Can you work these out from the model? Positions are in its coordinate system, mm. Face numbers are marked on the shaded views. Round coordinates to 2 decimals unless told otherwise and drop trailing zeros. Loops run counter-clockwise (first coordinate to the right, second up) from the corner with the lowest first, then second, coordinate; pieces in that order, holes last. Notation, with made-up numbers: (-35.75, -27.5) -> (-25.75, -27.5) arc R26 cw to (-25.75, -3.5) -> close; hole circle Ø7 at (-31, -4). An arc over 180 degrees is marked (long way). Use a Markdown table: item, result.
from build123d import *

# Parameters (mm, degrees)
BOSS_EXTRUDE1_DEPTH = 25
BOSS_EXTRUDE2_DEPTH = 15
CUT_EXTRUDE1_REACH  = 42.894
SKETCH3_R           = 1.5
CUT_EXTRUDE2_REACH  = 42.894
SKETCH4_R           = 1.6
CUT_EXTRUDE3_DEPTH  = 41.591655546


with BuildPart() as part:
    # Sketch1 → Boss-Extrude1 (new body)
    with BuildSketch(Plane.XY):
        Polygon((0, 0), (4.128054425, 7.15), (-4.6, 7.15), (-4.6, 5.15), (0.66395281, 5.15), (-1.732050808, 1), align=None)
    extrude(amount=BOSS_EXTRUDE1_DEPTH)

    # Sketch2 → Boss-Extrude2 (add)
    with BuildSketch(Plane.XY.offset(25)):
        Polygon((4.128054425, 7.15), (0, 0), (-1.732050808, 1), (1.818653348, 7.15), align=None)
    extrude(amount=BOSS_EXTRUDE2_DEPTH)

    # Sketch3 → Cut-Extrude1 (cut, up to next)
    with BuildSketch(Plane(origin=(0, 0, 0), x_dir=(0, 0, -1), z_dir=(0.8660254037844365, -0.5000000000000039, 0)), mode=Mode.PRIVATE) as cut_extrude1_sk1:
        with Locations(Location((-37.5, 2.5, 0), (0, 0, 90))):
            Circle(SKETCH3_R)
    cut_extrude1_tool1 = extrude(cut_extrude1_sk1.sketch, amount=-CUT_EXTRUDE1_REACH, mode=Mode.PRIVATE) & part.part
    # Sketch3 → Cut-Extrude1 (cut, up to next)
    with BuildSketch(Plane(origin=(0, 0, 0), x_dir=(0, 0, -1), z_dir=(0.8660254037844365, -0.5000000000000039, 0)), mode=Mode.PRIVATE) as cut_extrude1_sk2:
        with Locations(Location((-2.5, 2.5, 0), (0, 0, 90))):
            Circle(SKETCH3_R)
    cut_extrude1_tool2 = extrude(cut_extrude1_sk2.sketch, amount=-CUT_EXTRUDE1_REACH, mode=Mode.PRIVATE) & part.part
    add(cut_extrude1_tool1.solids().sort_by_distance((1.25, 2.165064, 37.5))[0], mode=Mode.SUBTRACT)
    add(cut_extrude1_tool2.solids().sort_by_distance((1.25, 2.165064, 2.5))[0], mode=Mode.SUBTRACT)

    # Sketch4 → Cut-Extrude2 (cut, up to next)
    with BuildSketch(Plane(origin=(0, 7.15, 0), x_dir=(1, 0, 0), z_dir=(0, 1, 0)), mode=Mode.PRIVATE) as cut_extrude2_sk1:
        with Locations(Location((-0.6, -8, 0), (0, 0, 180))):
            Circle(SKETCH4_R)
    cut_extrude2_tool1 = extrude(cut_extrude2_sk1.sketch, amount=-CUT_EXTRUDE2_REACH, mode=Mode.PRIVATE) & part.part
    # Sketch4 → Cut-Extrude2 (cut, up to next)
    with BuildSketch(Plane(origin=(0, 7.15, 0), x_dir=(1, 0, 0), z_dir=(0, 1, 0)), mode=Mode.PRIVATE) as cut_extrude2_sk2:
        with Locations(Location((-0.6, -20.5, 0), (0, 0, 180))):
            Circle(SKETCH4_R)
    cut_extrude2_tool2 = extrude(cut_extrude2_sk2.sketch, amount=-CUT_EXTRUDE2_REACH, mode=Mode.PRIVATE) & part.part
    add(cut_extrude2_tool1.solids().sort_by_distance((-0.6, 7.15, 8))[0], mode=Mode.SUBTRACT)
    add(cut_extrude2_tool2.solids().sort_by_distance((-0.6, 7.15, 20.5))[0], mode=Mode.SUBTRACT)

    # Sketch5 → Cut-Extrude3 (cut, through all)
    with BuildSketch(Plane.XZ.offset(-5.15)):
        with BuildLine():
            Line((-0.6, 23.5), (-3.6, 23.5))
            Line((-3.6, 23.5), (-3.6, 17.5))
            Line((-3.6, 17.5), (-0.6, 17.5))
            ThreePointArc((-0.6, 17.5), (2.4, 20.5), (-0.6, 23.5))
        make_face()
        with BuildLine():
            Line((-0.6, 11), (-3.6, 11))
            Line((-3.6, 11), (-3.6, 5))
            Line((-3.6, 5), (-0.6, 5))
            ThreePointArc((-0.6, 5), (2.4, 8), (-0.6, 11))
        make_face()
    extrude(amount=CUT_EXTRUDE3_DEPTH, mode=Mode.SUBTRACT)


solid = part.part
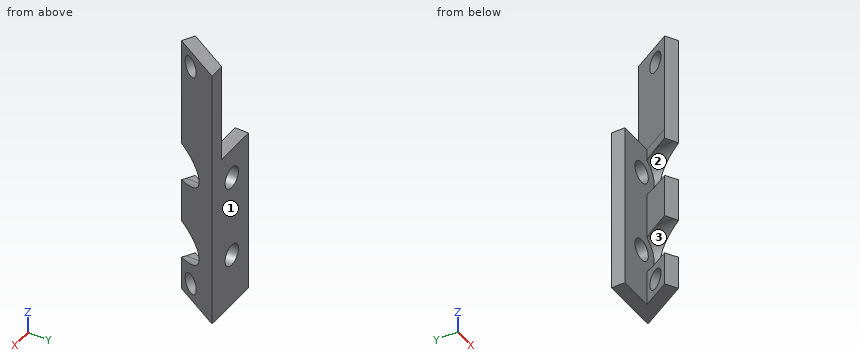
1. I want a section at A-A (z = 21). Please give me the cut outline in (x, y), plus the area to 3 significant figures.
Answer sheet:
| item | result |
|---|---|
| outline | (-4.6, 5.15) -> (-2.12, 5.15) -> (-2.12, 7.15) -> (-4.6, 7.15) -> close; (0.92, 5.15) -> (2.36, 5.15) -> (2.36, 4.08) -> (4.13, 7.15) -> (0.92, 7.15) -> close |
| area | 10.5 mm² |
2. I want a section at C-C (x = -3.5). Please give me the cut outline in (y, z), plus the area to 3 significant figures.
Answer sheet:
| item | result |
|---|---|
| outline | (5.15, 0) -> (7.15, 0) -> (7.15, 25) -> (5.15, 25) -> close |
| area | 50.0 mm² |
3. Will these pins go through, and if not, where does the flat tip stop? pin 1 Ø2 at (x, z) = (0.5, 6.5) entering from -Y; pin 2 Ø4 at (y, z) = (2.5, 15) entering from -X; pin 3 Ø1.5 at (x, z) = (-0.5, 32.5) entering from -Y.
Answer sheet:
| item | result |
|---|---|
| pin 1 | stops at y = 5.15 |
| pin 2 | stops at x = -1.73 |
| pin 3 | stops at y = 0 |
4. If we mould it in two halves opening along Z, with no side actions, what happens to the marked faces 1, 2 and 3? For each: +Z half, -Z half, draft (parallel to the pull), parting line (faces both ways), or undercut.
Answer sheet:
| item | result |
|---|---|
| face 1 | draft |
| face 2 | undercut |
| face 3 | undercut |
5. I want a section at D-D (z = 13). Please give me the cut outline in (x, y).
Answer sheet:
| item | result |
|---|---|
| outline | (-4.6, 5.15) -> (0.66, 5.15) -> (-1.73, 1) -> (0, 0) -> (4.13, 7.15) -> (-4.6, 7.15) -> close |
6. I want a section at B-B (y = 5.5). Please give me the cut outline in (x, z), plus the area to 3 significant figures.
Answer sheet:
| item | result |
|---|---|
| outline | (-4.6, 0) -> (3.18, 0) -> (3.18, 40) -> (0.87, 40) -> (0.87, 25) -> (-4.6, 25) -> close; hole circle Ø3.2 at (-0.6, 8); hole circle Ø3.2 at (-0.6, 20.5) |
| area | 213 mm² |
7. I need wall thicknesses on line 1 (Z direction, x = -0.6, y = 6.35); line 2 (Z direction, x = 0, y = 2); line 3 (Z direction, x = -2, y = 5.25). Which ranges of each line are inside material? Lowest first, please.
Answer sheet:
| item | result |
|---|---|
| line 1 | z = 0 to 6.4, 9.6 to 18.9, 22.1 to 25 |
| line 2 | z = 0 to 1.21, 3.79 to 5.06, 10.94 to 17.56, 23.44 to 36.21, 38.79 to 40 |
| line 3 | z = 0 to 7.23, 8.77 to 19.73, 21.27 to 25 |
